from build123d import *

# Parameters (mm, degrees)
SALIENTE_EXTRUIR1_DEPTH = 10
CROQUIS5_R              = 3
CORTAR_EXTRUIR1_DEPTH   = 169.229753611


with BuildPart() as part:
    # Barrer1: sweep along a path in Croquis3
    with BuildLine(Plane(origin=(0, 0, 0), x_dir=(1, 0, 0), z_dir=(0, 1, 0))) as barrer1_path:
        Line((0, 0), (0, -50))
        Line((0, -50), (159.5, -50))
        Line((159.5, -50), (159.5, 0))
    # Croquis1 → Barrer1 (sweep)
    with BuildSketch(Plane.XY):
        Polygon((0, 0), (0, 11.3), (13, 11.3), (13, 6.3), (5, 6.3), (5, 0), align=None)
    sweep(path=barrer1_path.line, transition=Transition.RIGHT)

    # Croquis4 → Saliente-Extruir1 (add)
    with BuildSketch(Plane.XY.offset(50)):
        with BuildLine():
            Line((13.25, 11.3), (23.25, 11.3))
            Line((23.25, 11.3), (23.25, 14))
            ThreePointArc((23.25, 14), (18.25, 19), (13.25, 14))
            Line((13.25, 14), (13.25, 11.3))
        make_face()
    saliente_extruir1 = extrude(amount=-SALIENTE_EXTRUIR1_DEPTH)

    # Croquis5 → Cortar-Extruir1 (cut, through all)
    with BuildSketch(Plane.XY.offset(50)):
        with Locations((18.25, 14)):
            Circle(CROQUIS5_R)
    cortar_extruir1 = extrude(amount=-CORTAR_EXTRUIR1_DEPTH, mode=Mode.SUBTRACT)

    # Simetría1: Saliente-Extruir1, Cortar-Extruir1 across plane
    add(saliente_extruir1.mirror(Plane(origin=(79.75, 0, 0), x_dir=(0, 0, 1), z_dir=(1, 0, 0))))
    add(cortar_extruir1.mirror(Plane(origin=(79.75, 0, 0), x_dir=(0, 0, 1), z_dir=(1, 0, 0))), mode=Mode.SUBTRACT)


solid = part.part
Read the model definition and answer for the solid it produces. Units are mm, in the model's axes. A direction names the side the tool comes from. Give positions to 0.01 mm unless a question says otherwise; leave off trailing zeros. Write each loop counter-clockwise with the first axis right and the second up, starting at its lowest first coordinate (ties: lowest second). Pieces come first, ordered by that corner, then holes. Notation, with made-up numbers: (28, 67) -> (35, 67) arc R26 cw to (35, 97) -> close; hole circle Ø8 at (-29, -15). An arc over 180 degrees is marked (long way). Answer as a JSON object with one key per item and string values. Group by question number.
1) Find section A-A (z = 17). Write down the section's boundary in (x, y), and give its area (3 significant figures).
2) Find section B-B (y = 8.5). Write down the section's boundary in (x, z).
3) Each of these flat-tipped pins is pushed along its axis until it touches: P1, Ø3, axis at y = 13, z = 46.5, coming from the +X side; P2, Ø4, axis at x = 88, y = 8.5, coming from the -Z side; P3, Ø1.5, axis at x = 32.5, y = 3, coming from the -Z side. Where does it stop, or does it pass through?
4) Consider L1, parallel to X at y = 14, z = 45.75; L2, parallel to Y at x = 18.25, z = 44.25; L3, parallel to Y at x = 141, z = 47. Determine where each line is inside the solid, lowest interval first. Write a range as from..to.
5) Find section D-D (x = 64.5). Write down the section's boundary in (y, z), and give its area (3 significant figures).
6) A tool of negligible diameter and unlimited length cuts with its end or side. For faces 5 (the flat face through (23.25, 13, 45)), 6 (the flat face through (81, 9, 37)), 7 (the flat face through (140, 17, 40)), 8 (the flat face through (5, 3, 23)), from which of +Z, -Z, +X, -X, +Y, -Y can it reach the whole face along a straight path? Write none if from no direction.
7) The mould has two halves that part along X. Classify faces 1 (the flat face through (13.25, 13, 45)), 2 (the flat face through (81, 3, 45)), 3 (the flat face through (146.25, 13, 45)), 4 (the flat face through (79.4, 0, 45.5)): +X half, -X half, draft (parallel to the pull), parting line (faces both ways), or undercut.
8) Find section C-C (x = 11.5). Write down the section's boundary in (y, z).
Values follow:
{
 "1": {"outline": "(0, 0) -> (5, 0) -> (5, 6.3) -> (13, 6.3) -> (13, 11.3) -> (0, 11.3) -> close; (146.5, 6.3) -> (154.5, 6.3) -> (154.5, 0) -> (159.5, 0) -> (159.5, 11.3) -> (146.5, 11.3) -> close", "area": "193 mm2"},
 "2": {"outline": "(0, 0) -> (13, 0) -> (13, 37) -> (146.5, 37) -> (146.5, 0) -> (159.5, 0) -> (159.5, 50) -> (0, 50) -> close"},
 "3": {"P1": "stops at x = 146.25", "P2": "stops at z = 37", "P3": "stops at z = 45"},
 "4": {"L1": "x = 13.25..15.25, 21.25..23.25, 136.25..138.25, 144.25..146.25", "L2": "y = 6.3..11, 17..19", "L3": "y = 0..11.01, 16.99..18.99"},
 "5": {"outline": "(0, 45) -> (6.3, 45) -> (6.3, 37) -> (11.3, 37) -> (11.3, 50) -> (0, 50) -> close", "area": "96.5 mm2"},
 "6": {"face 5": "+Z, -Z, +Y", "face 6": "-Z, +Y, -Y", "face 7": "-Z, +X, -X, +Y", "face 8": "-Z, -Y"},
 "7": {"face 1": "-X half", "face 2": "undercut", "face 3": "+X half", "face 4": "draft"},
 "8": {"outline": "(0, 45) -> (6.3, 45) -> (6.3, 0) -> (11.3, 0) -> (11.3, 50) -> (0, 50) -> close"}
}
